from build123d import *

# Parameters (mm, degrees)
F0_W     = 15
F0_H     = 25
F1_DEPTH = 3
F2_R     = 3
F3_DEPTH = 50


# Not quite as in the source:
# - a feature names something its author has since deleted; it is built from what else it names


with BuildPart() as f1:
    # F0 (on Top) → F1 (new body)
    with BuildSketch(Plane.XY):
        Rectangle(F0_W, F0_H)
    extrude(amount=F1_DEPTH)

    # F2 (on Top) → F3 (join)
    with BuildSketch(Plane.XY):
        Circle(F2_R)
    extrude(amount=F3_DEPTH)


solid = f1.part
The listing builds one solid part. Answer for the finished solid, in the listing's coordinates (mm). A direction names the side the tool comes from. Round coordinates to 2 decimals unless told otherwise and drop trailing zeros. Order: outer loops, then holes, each group sorted by start corner. A loop starts at its lowest first (then second) coordinate and runs counter-clockwise, first axis right, second up. Notation, with made-up numbers: (-12.75, 80.25) -> (8.25, 80.25) arc R13 ccw to (8.25, 90.25) -> close; hole circle Ø5 at (-36.75, 15). An arc over 180 degrees is marked (long way). One line per item, written item: value.
Item 1: For faces 1 (the flat face through (0, -12.5, 1)), 2 (the flat face through (-2, 3, 3)), determine the directions among +Z, -Z, +X, -X, +Y, -Y from which every point of the face is accessible in a straight line to the end or side of a thin tool.
Taken from the geometry:
face 1: +Z, -Z, +X, -X, -Y
face 2: +Z
Item 2: Find section A-A, the plane x = 0. Give the vertices of the cut face in (y, z), then the cut area to 3 significant figures.
Taken from the geometry:
outline: (-12.5, 0) -> (12.5, 0) -> (12.5, 3) -> (3, 3) -> (3, 50) -> (-3, 50) -> (-3, 3) -> (-12.5, 3) -> close
area: 357 mm2
Item 3: Straight lines are drawn through the part: L1, parallel to Z at x = -2.5, y = -9.75; L2, parallel to Y at x = 0, z = 23; L3, parallel to Y at x = -1, z = 48.5. For each, find the intervals that lie inside material, in ascending order.
Taken from the geometry:
L1: z = 0 to 3
L2: y = -3 to 3
L3: y = -2.83 to 2.83
Item 4: Find section B-B, the plane y = 0. Give the vertices of the cut face in (x, z).
Taken from the geometry:
outline: (-7.5, 0) -> (7.5, 0) -> (7.5, 3) -> (3, 3) -> (3, 50) -> (-3, 50) -> (-3, 3) -> (-7.5, 3) -> close
Item 5: Given P1, Ø12, axis at y = -2, z = 11.5, coming from the -X side; P2, Ø8, axis at x = -3, z = 39.5, coming from the +Y side; P3, Ø10, axis at y = 9.5, z = 21.5, coming from the +X side, each flat-ended and moving along its own axis, determine where each tip first touches the part or whether it passes through.
Taken from the geometry:
P1: stops at x = -3
P2: stops at y = 3
P3: passes through
Item 6: Find section C-C, the plane z = 28.5. Give the vertices of the cut face in (x, y), then the cut area to 3 significant figures.
Taken from the geometry:
outline: circle Ø6 at (0, 0)
area: 28.3 mm2
Item 7: Find section D-D, the plane x = 6. Give the vertices of the cut face in (y, z), then the cut area to 3 significant figures.
Taken from the geometry:
outline: (-12.5, 0) -> (12.5, 0) -> (12.5, 3) -> (-12.5, 3) -> close
area: 75.0 mm2
